Geometry check sheet. Reference: the model listing, model coordinates, mm. A direction names the side the tool comes from. Round coordinates to 2 decimals unless told otherwise and drop trailing zeros. Write each loop counter-clockwise with the first axis right and the second up, starting at its lowest first coordinate (ties: lowest second). Pieces come first, ordered by that corner, then holes.
Item 1: Cross-section at D-D (x = 21.5). Enter the section's corners in (y, z).
Item 2: Cross-section at B-B (z = -56.55). Enter the section's corners in (x, y).
Item 3: Cross-section at A-A (y = 0.5). Enter the section's corners in (x, z).
Item 4: Draft check along Y on faces 1 (the face through (-33, 0, -66.55)), 2 (the face through (-33.18, 0.57, -58.1)), 3 (the face through (-32, 8.15, -21)), 4 (the face through (-33.178, -0.094, -17.318)). Enter one of: pulls with the +Y half, pulls with the -Y half, needs draft (parallel to the pull), parting line crosses it, or undercut.
Item 5: Depth check by flat-ended pin: P1, Ø5, axis at y = 0.5, z = -18.75, coming from the +X side; P2, Ø3, axis at y = 0.5, z = -56.55, coming from the +X side; P3, Ø2, axis at x = -5, y = -6.5, coming from the -Z side. Enter the tip coordinate at first touch or a pass-through.
Item 6: Access from +Z, -Z, +X, -X, +Y, -Y to the whole of each face (thin tool, end or side, straight path). Record for faces 5 (the face through (27.263, 0, 2)), 6 (the face through (-2, 0, 0)).
Item 7: Cross-section at C-C (y = 6.25). Enter the section's corners in (x, z).
Item 8: Scan lines: probe 1 along Y at (x, z) = (-33, -56.55); probe 2 along Z at (x, y) = (-13, 4); probe 3 along X at (y, z) = (-3.75, -17.5). Record each from-to range of solid material in increasing order.
from build123d import *

# Parameters (mm, degrees)
SKETCH_1_W      = 62.4134
SKETCH_1_H      = 16.3
EXTRUDE_1_DEPTH = 4
SKETCH_3_W      = 70.55
SKETCH_3_H      = 16.3
SKETCH_3_R      = 1.55
EXTRUDE_3_DEPTH = 4


with BuildPart() as part:
    # 草图1 → 凸台-拉伸1 (new body)
    with BuildSketch(Plane.XY):
        with Locations((-3.9433, 0)):
            Rectangle(SKETCH_1_W, SKETCH_1_H)
    extrude(amount=EXTRUDE_1_DEPTH)

    # 草图3 → 凸台-拉伸3 (add)
    with BuildSketch(Plane.ZY.offset(35.15)):
        with Locations((-31.275, 0)):
            Rectangle(SKETCH_3_W, SKETCH_3_H)
        with Locations((-56.55, 0.5)):
            Circle(SKETCH_3_R, mode=Mode.SUBTRACT)
        with Locations((-18.75, 0.5)):
            Circle(SKETCH_3_R, mode=Mode.SUBTRACT)
    extrude(amount=-EXTRUDE_3_DEPTH)


solid = part.part
Resolved:
1. outline: (-8.15, 0) - (8.15, 0) - (8.15, 4) - (-8.15, 4) - close
2. outline: (-35.15, -8.15) - (-31.15, -8.15) - (-31.15, -1.05) - (-35.15, -1.05) - close; (-35.15, 2.05) - (-31.15, 2.05) - (-31.15, 8.15) - (-35.15, 8.15) - close
3. outline: (-35.15, -66.55) - (-31.15, -66.55) - (-31.15, -58.1) - (-35.15, -58.1) - close; (-35.15, -55) - (-31.15, -55) - (-31.15, -20.3) - (-35.15, -20.3) - close; (-35.15, -17.2) - (-31.15, -17.2) - (-31.15, 0) - (27.26, 0) - (27.26, 4) - (-35.15, 4) - close
4. face 1: needs draft
4. face 2: undercut
4. face 3: pulls with the +Y half
4. face 4: undercut
5. P1: stops at x = -31.15
5. P2: passes through
5. P3: stops at z = 0
6. face 5: +Z, -Z, +X, +Y, -Y
6. face 6: -Z, +X, +Y, -Y
7. outline: (-35.15, -66.55) - (-31.15, -66.55) - (-31.15, 0) - (27.26, 0) - (27.26, 4) - (-35.15, 4) - close
8. probe 1: y = -8.15 to -1.05, 2.05 to 8.15
8. probe 2: z = 0 to 4
8. probe 3: x = -35.15 to -31.15
